The model under review builds one solid part; all positions refer to its coordinate system, in mm. Round coordinates to 2 decimals unless told otherwise and drop trailing zeros. Loops run counter-clockwise (first coordinate to the right, second up) from the corner with the lowest first, then second, coordinate; pieces in that order, holes last. Notation, with made-up numbers: (77.5, -18) - (102.5, -18) arc R20 ccw to (102.5, 10) - close; hole circle Ø7 at (-34, 86.5). An arc over 180 degrees is marked (long way). Answer as CSV lines item,"result".
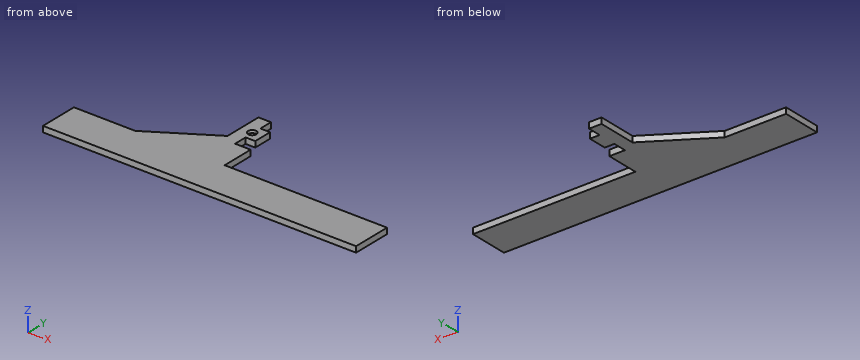
from build123d import *

# Parameters (mm, degrees)
SALIENTE_EXTRUIR1_DEPTH = 15
CROQUIS4_R              = 11
CORTAR_EXTRUIR1_DEPTH   = 7


with BuildPart() as part:
    # Croquis1 → Saliente-Extruir1 (new body)
    with BuildSketch(Plane.XY):
        Polygon((-15, 50), (-15, 134), (-55, 134), (-55, 168), (-30, 168), (-30, 216), (-55, 216), (-55, 250), (-87.48, 250), (-87.48, 150), (-246.54, 50), (-405.6, 50), (-405.6, -50), (405.6, -50), (405.6, 50), align=None)
    extrude(amount=SALIENTE_EXTRUIR1_DEPTH)

    # Croquis4 → Cortar-Extruir1 (cut)
    with BuildSketch(Plane.XY.offset(15)):
        with Locations((-56.98, 192)):
            Circle(CROQUIS4_R)
    extrude(amount=-CORTAR_EXTRUIR1_DEPTH, mode=Mode.SUBTRACT)


solid = part.part
1. Clearance check with flat-ended pins moving along their axes: pin 1 (7.5 mm diameter, centred on x = -34, z = 9.5, fed in from +Y); pin 2 (6.5 mm diameter, centred on x = -52.5, y = 193.5, fed in from +Z); pin 3 (4.5 mm diameter, centred on y = 236, z = 5.5, fed in from +X). State where each tip first meets the part, or that it passes through.
Numbers:
pin 1,"stops at y = 216"
pin 2,"stops at z = 8"
pin 3,"stops at x = -55"
2. Take a section at C-C (x = 62). State the section outline as (y, z) points.
Numbers:
outline,"(-50, 0) - (50, 0) - (50, 15) - (-50, 15) - close"
3. Take a section at B-B (y = 192). State the section outline as (x, z) points, plus the area to 3 significant figures.
Numbers:
outline,"(-87.48, 0) - (-30, 0) - (-30, 15) - (-45.98, 15) - (-45.98, 8) - (-67.98, 8) - (-67.98, 15) - (-87.48, 15) - close"
area,"708 mm²"
4. Wall thickness on probe 1 along Y at (x, z) = (-56.98, 10.5); probe 2 along X at (y, z) = (225, 2); probe 3 along Y at (x, z) = (103.5, 9): over which ranges is each line inside the solid? List them lowest first.
Numbers:
probe 1,"y = -50 to 181, 203 to 250"
probe 2,"x = -87.48 to -55"
probe 3,"y = -50 to 50"
5. Take a section at A-A (z = 11.5). State the section outline as (x, y) points.
Numbers:
outline,"(-405.6, -50) - (405.6, -50) - (405.6, 50) - (-15, 50) - (-15, 134) - (-55, 134) - (-55, 168) - (-30, 168) - (-30, 216) - (-55, 216) - (-55, 250) - (-87.48, 250) - (-87.48, 150) - (-246.54, 50) - (-405.6, 50) - close; hole circle Ø22 at (-56.98, 192)"
